Can you work these out from the model? Positions are in its coordinate system, mm. Face numbers are marked on the shaded views. A direction names the side the tool comes from. Coordinates: 2 decimals unless noted, no trailing zeros. Loops run counter-clockwise (first coordinate to the right, second up) from the corner with the lowest first, then second, coordinate; pieces in that order, holes last.
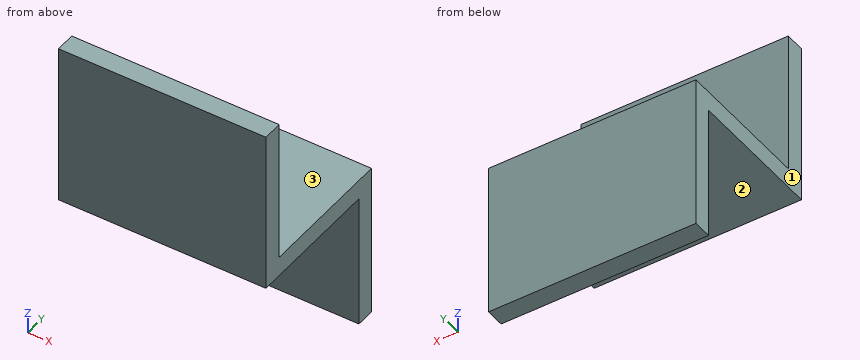
```python
from build123d import *

# Parameters (mm, degrees)
EXTRUDE4_DEPTH = 66.294


with BuildPart() as part:
    # Sketch10 → Extrude4 (new body)
    with BuildSketch(Plane(origin=(0, 0, 0), x_dir=(0, 0, -1), z_dir=(1, 0, 0))):
        Polygon((52.353300196, 44.627176404), (52.353300196, 0), (0, 0), (0, 6.35), (46.003300196, 6.35), (46.003300196, 50.658753449), (52.353300196, 50.658753449), (95.762817201, 50.658753449), (95.762817201, 44.627176404), align=None)
    extrude(amount=-EXTRUDE4_DEPTH)


solid = part.part
```
(1) If I drill on probe 1 along Z at (x, y) = (-46, 38); probe 2 along Y at (x, z) = (-11.5, -52.5); probe 3 along Z at (x, y) = (-30.5, 48.5), over which ranges is the centre line in solid material (lowest first)?
Check values:
probe 1: z = -52.35 to -46
probe 2: y = 44.63 to 50.66
probe 3: z = -95.76 to -46
(2) I want a section at C-C on y = 18.5. Write out the boundary of the cut face in (x, z), then the cut area to 3 significant figures.
Check values:
outline: (-66.29, -52.35) - (0, -52.35) - (0, -46) - (-66.29, -46) - close
area: 421 mm2
(3) I'm going to push flat-ended pins straight in: pin 1 (1 mm diameter, centred on x = -45, y = 9.5, fed in from -Z); pin 2 (5 mm diameter, centred on x = -45, z = -41, fed in from +Y); pin 3 (10 mm diameter, centred on x = -55.5, y = 32, fed in from +Z). Where does each tip first touch, or does it pass through?
Check values:
pin 1: stops at z = -52.35
pin 2: stops at y = 6.35
pin 3: stops at z = -46
(4) Which directions (+Z, -Z, +X, -X, +Y, -Y) give clear straight access to the entire face, cutting with the end or side of a thin tool? Please do the marked faces 1, 2 and 3.
Check values:
face 1: +Z, -Z, -X, +Y, -Y
face 2: -Z, +X, -X, -Y
face 3: +Z, +X, -X, +Y
(5) I want a section at B-B on z = -25.5. Write out the boundary of the cut face in (x, y).
Check values:
outline: (-66.29, 0) - (0, 0) - (0, 6.35) - (-66.29, 6.35) - close
(6) I want a section at A-A on x = -26.5. Write out the boundary of the cut face in (y, z).
Check values:
outline: (0, -52.35) - (44.63, -52.35) - (44.63, -95.76) - (50.66, -95.76) - (50.66, -46) - (6.35, -46) - (6.35, 0) - (0, 0) - close
